Input: part model. Units: mm. Frame: model coordinates. A direction names the side the tool comes from. Coordinates: 2 decimals unless noted, no trailing zeros. Loops run counter-clockwise (first coordinate to the right, second up) from the corner with the lowest first, then second, coordinate; pieces in that order, holes last.
(1) Line query: L1, parallel to Y at x = 30, z = 4.7; L2, parallel to Y at x = -10, z = 1.05; L3, parallel to X at y = -1.75, z = 4.75. Output: solid intervals per line, ascending.
(2) Section D-D, the plane z = 5.25. Return loops of the section in (x, y), then the cut area to 3 significant figures.
(3) Mould query, pull axis X, two halves, no side actions, for faces 3 (the face through (-38, 19, 4)), 4 (the face through (-12.854, -0.676, 3.451)), 5 (the face through (40, 8, 3)). Classes: released by +X, released by -X, zero draft, split by the parting line, or undercut.
(4) Section C-C, the plane y = 10. Give the number of separate pieces and of enclosed holes in the cut face, then the cut area to 4 significant figures.
(5) Section A-A, the plane z = 1.5. Return loops of the section in (x, y), then the cut area to 3 significant figures.
(6) Section B-B, the plane x = -30. Return loops of the section in (y, z).
(7) Set-up query: faces 1 (the face through (-38.319, 18.246, 6.858)), 2 (the face through (32.2, 7.8, 3)). Return all of +Z, -Z, +X, -X, +Y, -Y with unobstructed straight access to the full face (end or side cutting, diameter ignored); none if empty.
Autodesk Fusion 360 part; units mm, degrees
sketch "Skizze1" plane through (0, 0, 0) normal (0, 0, 1) x (1, 0, 0)
  circle A0 centre (-15, 0) radius 2.25
  circle A1 centre (-30, 10) radius 2.75
  line L0 (-40, 20) -> (0, 20)
  line L1 (0, 20) -> (0, -5)
  line L2 (0, -5) -> (-40, -5)
  line L3 (-40, -5) -> (-40, 20)
  circle A2 centre (-10, 10) radius 2.75
  line L4 (-30, 10) -> (0, 10)
  circle A3 centre (-10, 10) radius 5
  circle A4 centre (-30, 10) radius 5
  line L5 (-15, 0) -> (0, 0)
  dimension "d1" = 4.5
  dimension "d2" = 15
  dimension "d4" = 5.5
  dimension "d5" = 40
  dimension "d16" = 30
  dimension "d17" = 20
  dimension "d18" = 10
  dimension "d19" = 10
  dimension "d20" = 10
  dimension "d21" = 5
extrude "Extrusion1" add sketch "Skizze1" along normal blind 7 contours L0 L1 L2 L3
extrude "Extrusion2" add sketch "Skizze1" along normal blind 3 contours A4 | A2 L4 A3 | A2 L4 A3
fillet "Abrundung1" radius 5 2 edges at (-40, 20, 3.5) (-40, -5, 3.5)
mirror "Spiegeln1" about plane through (0, 20, 0) normal (1, 0, 0) of bodies 1 merged
chamfer "Fase1" distance 0.5 angle 45 16 edges at (0, 20, 7) (38.5355, 18.5355, 7) (40, 7.5, 7) (38.5355, -3.5355, 7) (0, -5, 7) (-38.5355, -3.5355, 7) (-40, 7.5, 7) (-38.5355, 18.5355, 7) (0, -5, 0) (-38.5355, -3.5355, 0) (-40, 7.5, 0) (-38.5355, 18.5355, 0) (0, 20, 0) (38.5355, 18.5355, 0) (40, 7.5, 0) (38.5355, -3.5355, 0)
equation "d2 = ( 30 / 2 ) * 1 mm"
equation "d5 = ( 80 / 2 ) * 1 mm"
equation "d16 = ( 80 / 2 ) * 1 mm - 10 mm"
Report:
1. L1: y = -5 to 5, 15 to 20
1. L2: y = -5 to 7.25, 12.75 to 20
1. L3: x = -39.68 to -16.41, -13.59 to 13.59, 16.41 to 39.68
2. outline: (-40, 0) arc R5 ccw to (-35, -5) - (35, -5) arc R5 ccw to (40, 0) - (40, 15) arc R5 ccw to (35, 20) - (-35, 20) arc R5 ccw to (-40, 15) - close; hole circle Ø10 at (-30, 10); hole circle Ø4.5 at (-15, 0); hole circle Ø10 at (-10, 10); hole circle Ø10 at (10, 10); hole circle Ø4.5 at (15, 0); hole circle Ø10 at (30, 10)
2. area: 1,630 mm2
3. face 3: released by -X
3. face 4: undercut
3. face 5: released by +X
4. separate pieces: 5
4. enclosed holes: 0
4. area: 333.5 mm2
5. outline: (-40, 0) arc R5 ccw to (-35, -5) - (35, -5) arc R5 ccw to (40, 0) - (40, 15) arc R5 ccw to (35, 20) - (-35, 20) arc R5 ccw to (-40, 15) - close; hole circle Ø5.5 at (-30, 10); hole circle Ø4.5 at (-15, 0); hole circle Ø5.5 at (-10, 10); hole circle Ø5.5 at (10, 10); hole circle Ø4.5 at (15, 0); hole circle Ø5.5 at (30, 10)
5. area: 1,850 mm2
6. outline: (-5, 0.5) - (-4.5, 0) - (7.25, 0) - (7.25, 3) - (5, 3) - (5, 7) - (-4.5, 7) - (-5, 6.5) - close; (12.75, 0) - (19.5, 0) - (20, 0.5) - (20, 6.5) - (19.5, 7) - (15, 7) - (15, 3) - (12.75, 3) - close
7. face 1: +Z, -X, +Y
7. face 2: +Z
